Job drawing, mm, ordinate dimensions from the low corner. One solid piece. Give positions to 0.01 mm unless a question says otherwise; leave off trailing zeros. Loops run counter-clockwise (first coordinate to the right, second up) from the corner with the lowest first, then second, coordinate; pieces in that order, holes last. Notation, with made-up numbers: M 14,23 L 40,23 A13 ccw 40,36 Z; hole C 83,45 d9. An arc over 180 degrees is marked long. One line per question, with ' | ' between items.
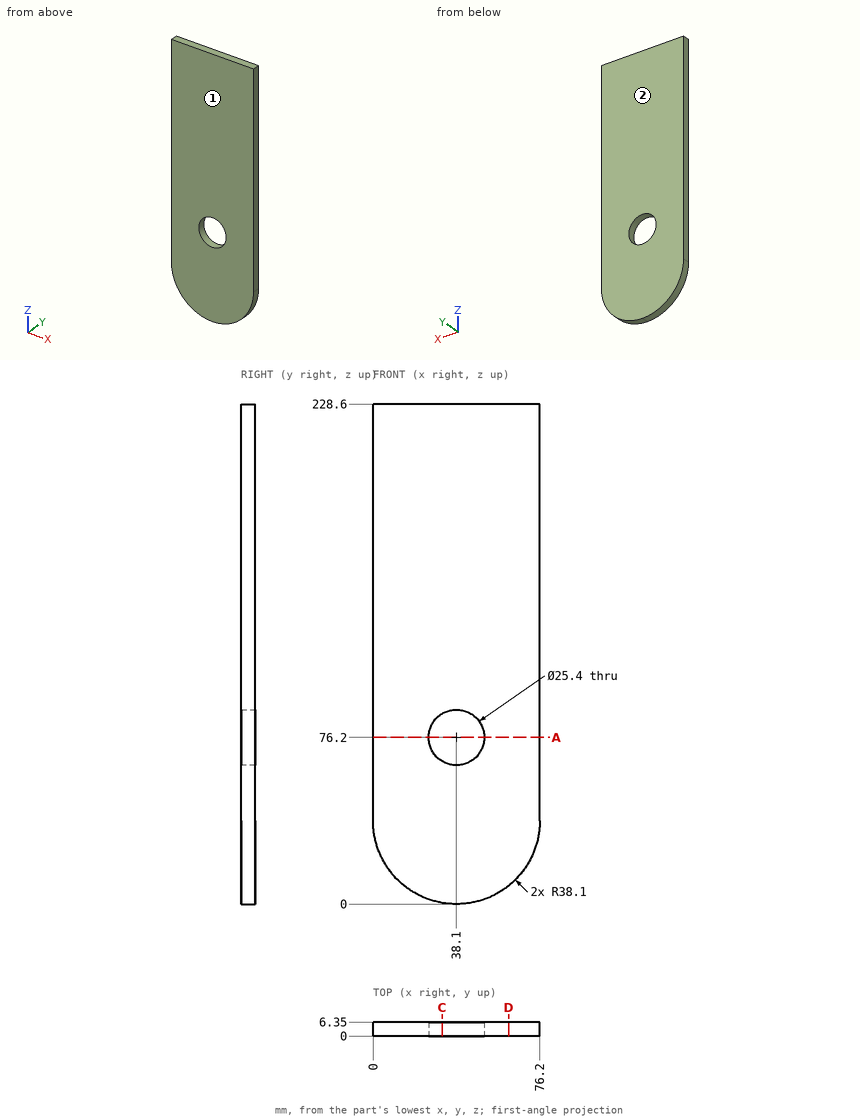
Item 1: Drill centre lines: line 1 along Z through (x, y) = (39, 1.25); line 2 along X through (y, z) = (2.25, 76.2); line 3 along Z through (x, y) = (13, 0.5). Where is each one in solid material? Low to high. Write a range as [from, to].
Conclusion:
line 1: [0.01, 63.53], [88.87, 228.6] | line 2: [0, 25.4], [50.8, 76.2] | line 3: [9.44, 228.6]
Item 2: Mould opens along Y. For the marked faces 1 and 2 say: pulls with the +Y half, pulls with the -Y half, needs draft (parallel to the pull), parting line crosses it, or undercut.
Conclusion:
face 1: pulls with the -Y half | face 2: pulls with the +Y half
Item 3: Saw through at A-A on z = 76.2. Give the cut face in (x, y).
Conclusion:
outline: M 0,0 L 25.4,0 L 25.4,6.35 L 0,6.35 Z; M 50.8,0 L 76.2,0 L 76.2,6.35 L 50.8,6.35 Z
Item 4: Saw through at C-C on x = 31.5. Give the cut face in (y, z).
Conclusion:
outline: M 0,0.58 L 6.35,0.58 L 6.35,65.35 L 0,65.35 Z; M 0,87.05 L 6.35,87.05 L 6.35,228.6 L 0,228.6 Z
Item 5: Saw through at D-D on x = 62. Give the cut face in (y, z).
Conclusion:
outline: M 0,8.43 L 6.35,8.43 L 6.35,228.6 L 0,228.6 Z
